Could you check a few things on this model? Use its own coordinates, in mm. A direction names the side the tool comes from. Give positions to 0.01 mm unless a question says otherwise; leave off trailing zeros. Loops run counter-clockwise (first coordinate to the right, second up) from the corner with the lowest first, then second, coordinate; pieces in that order, holes last. Notation, with made-up numbers: (-10.5, 26) - (4.5, 26) arc R27 cw to (4.5, 45) - close; hole circle Ø4 at (40.25, 62.5). An arc over 180 degrees is marked (long way). Write each question's results on one line, items separated by ' | '. Start each with the question number.
```python
from build123d import *

# Parameters (mm, degrees)
F1_DEPTH = 76.2
F4_D     = 4.318
F4_DEPTH = 12.7
F4_TIP   = 1.2972580765
F5_R     = 3.4925
F5_R_2   = 2.159
F6_DEPTH = 2.032


with BuildPart() as f1:
    # F0 (on Front) → F1 (new body)
    with BuildSketch(Plane.XZ):
        Polygon((0, 63.5), (0, 0), (9.525, 0), (9.525, 10.16), (6.985, 12.7), (6.985, 22.86), (9.525, 25.4), (9.525, 38.1), (6.985, 40.64), (6.985, 50.8), (9.525, 53.34), (9.525, 63.5), align=None)
    extrude(amount=F1_DEPTH)

    # F4
    with Locations(Plane.YZ.offset(9.525)):
        with Locations((-63.5, 58.42), (-12.7, 58.42), (-63.5, 5.08), (-12.7, 5.08)):
            Hole(F4_D / 2, depth=F4_DEPTH)
            with Locations((0, 0, -(F4_DEPTH + F4_TIP / 2))):  # 118° drill point
                Cone(0, F4_D / 2, F4_TIP, mode=Mode.SUBTRACT)

    # F5 (on face) → F6 (cut)
    with BuildSketch(Plane.YZ.offset(9.525)):
        with Locations((-63.5, 58.42)):
            Circle(F5_R)
        with Locations((-12.7, 58.42)):
            Circle(F5_R)
        with Locations((-63.5, 5.08)):
            Circle(F5_R)
        with Locations((-63.5, 5.08)):
            Circle(F5_R_2, mode=Mode.SUBTRACT)
        with Locations((-12.7, 5.08)):
            Circle(F5_R)
        with Locations((-12.7, 5.08)):
            Circle(F5_R_2, mode=Mode.SUBTRACT)
    extrude(amount=-F6_DEPTH, mode=Mode.SUBTRACT)


solid = f1.part
```
Q1. If we mould it in two halves opening along Z, with no side actions, what happens to faces 1 (the face through (5, -38, 0)), 2 (the face through (6.985, -38, 18)), 3 (the face through (5, -38, 63.5)), 4 (the face through (9.525, -38, 58))? For each: +Z half, -Z half, draft (parallel to the pull), parting line (faces both ways), or undercut.
Q2. I need wall thicknesses on L1, parallel to Z at x = 2.25, y = -63.5; L2, parallel to Y at x = 1.5, z = 5.08; L3, parallel to Y at x = 4, z = 60. Which ranges of each line are inside material? Lowest first, please. Write a range as from..to.
Q3. I want a section at C-C, the plane y = -33. List the corners of the cut face in (x, z) for me (3 decimals), then the cut area to 3 significant figures.
Q4. I want a section at D-D, the plane z = 47. List the corners of the cut face in (x, y) for me (3 decimals).
Q5. I want a section at A-A, the plane y = -63.5. List the corners of the cut face in (x, z) for me (1 decimal), then the cut area to 3 significant figures.
Q6. I'm going to push flat-ended pins straight in: pin 1 Ø5 at (y, z) = (-22, 17) entering from +X (3 decimals); pin 2 Ø2 at (y, z) = (-11.5, 4) entering from +X. Where does each tip first touch, or does it pass through?
Q7. I want a section at B-B, the plane z = 5.08. List the corners of the cut face in (x, y) for me (1 decimal).
Q8. Which directions (+Z, -Z, +X, -X, +Y, -Y) give clear straight access to the entire face, cutting with the end or side of a thin tool? Please do faces 5 (the face through (8.237, -37.567, 52.052)), 6 (the face through (0, -38, 32)), 7 (the face through (7.493, -64, 56)).
Conclusion:
1) face 1: -Z half | face 2: undercut | face 3: +Z half | face 4: draft
2) L1: 0..2.92, 7.24..56.26, 60.58..63.5 | L2: -76.2..-65.66, -61.34..-14.86, -10.54..0 | L3: -76.2..-64.97, -62.03..-14.17, -11.23..0
3) outline: (0, 0) - (9.525, 0) - (9.525, 10.16) - (6.985, 12.7) - (6.985, 22.86) - (9.525, 25.4) - (9.525, 38.1) - (6.985, 40.64) - (6.985, 50.8) - (9.525, 53.34) - (9.525, 63.5) - (0, 63.5) - close | area: 540 mm^2
4) outline: (0, -76.2) - (6.985, -76.2) - (6.985, 0) - (0, 0) - close
5) outline: (0, 0) - (9.5, 0) - (9.5, 1.6) - (7.5, 1.6) - (7.5, 2.9) - (0, 2.9) - close; (0, 7.2) - (7.5, 7.2) - (7.5, 8.6) - (9.5, 8.6) - (9.5, 10.2) - (7, 12.7) - (7, 22.9) - (9.5, 25.4) - (9.5, 38.1) - (7, 40.6) - (7, 50.8) - (9.5, 53.3) - (9.5, 54.9) - (7.5, 54.9) - (7.5, 56.3) - (0, 56.3) - close; (0, 60.6) - (7.5, 60.6) - (7.5, 61.9) - (9.5, 61.9) - (9.5, 63.5) - (0, 63.5) - close | area: 447 mm^2
6) pin 1: x = 6.985 | pin 2: x = 7.49
7) outline: (0, -76.2) - (9.5, -76.2) - (9.5, -67) - (7.5, -67) - (7.5, -65.7) - (0, -65.7) - close; (0, -61.3) - (7.5, -61.3) - (7.5, -60) - (9.5, -60) - (9.5, -16.2) - (7.5, -16.2) - (7.5, -14.9) - (0, -14.9) - close; (0, -10.5) - (7.5, -10.5) - (7.5, -9.2) - (9.5, -9.2) - (9.5, 0) - (0, 0) - close
8) face 5: +X, +Y, -Y | face 6: +Z, -Z, -X, +Y, -Y | face 7: +X
